Autodesk Inventor part; units mm, degrees
ref_plane "YZ Plane" through (0, 0, 0) normal (1, 0, 0) x (0, 1, 0)
ref_plane "XZ Plane" through (0, 0, 0) normal (0, 1, 0) x (-1, 0, 0)
ref_plane "XY Plane" through (0, 0, 0) normal (0, 0, 1) x (1, 0, 0)
sketch "スケッチ1" plane through (0, 0, 0) normal (0, 0, 1) x (1, 0, 0)
  line L0 (-25, -71.3) -> (25, -71.3)
  line L1 (25, -71.3) -> (25, 25)
  line L2 (25, 25) -> (-25, 25)
  line L3 (-25, 25) -> (-25, -71.3)
  line L4 (-25, -71.3) -> (25, 25) construction
  line L5 (25, -71.3) -> (-25, 25) construction
  circle A0 centre (0, 0) radius 19 construction
  point P0 (0, -23.15)
  point P1 (0, -23.15)
  dimension "d0" = 38
  dimension "d1" = 50
  dimension "d2" = 25
  dimension "d3" = 71.3
extrude "プレート1" add sketch "スケッチ1" along normal blind 2.3
sketch "スケッチ9" plane through (25, -69, 0) normal (0, -1, 0) x (1, 0, 0)
  line L0 (-50, 0) -> (0, 0)
  line L1 (0, 0) -> (0, 14.6)
  line L2 (0, 14.6) -> (-50, 14.6)
  line L3 (-50, 14.6) -> (-50, 0)
edge flange "フランジ3" height 14.6 angle 90 thickness 2.3 bend radius 2.3 thickness toward (0, -1, 0) relief tear relief width 2.3 relief depth 1.15 edges at (0, -71.3, 2.3) wall of the first edge with corners at (-25, -69, 0) (25, -69, 0) (25, -69, 14.6) (-25, -69, 14.6)
bend "曲げ3"
corner "コーナー3"
fillet "コーナーR1" radius 5 2 edges at (25, -70.15, 14.6) (-25, -70.15, 14.6)
sketch "スケッチ4" plane through (0, 0, 2.3) normal (0, 0, 1) x (1, 0, 0)
  circle A0 centre (0, 0) radius 15
  point P0 (0, 15)
  point P1 (-15, 0)
  point P2 (0, -15)
  point P3 (15, 0)
  dimension "d26" = 30
  dimension "d29" = 360
hole "穴1" at (0, 15, 2.3) at (-15, 0, 2.3) at (0, -15, 2.3) at (15, 0, 2.3) direction (0, 0, -1) diameter 3.2 end through all
sketch "スケッチ5" plane through (0, 0, 2.3) normal (0, 0, 1) x (1, 0, 0)
  circle A0 centre (0, 0) radius 16
  point P0 (-11.3137, 11.3137)
  point P1 (-11.3137, -11.3137)
  point P2 (11.3137, -11.3137)
  point P3 (11.3137, 11.3137)
  dimension "d38" = 32
  dimension "d41" = 360
hole "穴2" at (-11.3137, 11.3137, 2.3) at (-11.3137, -11.3137, 2.3) at (11.3137, -11.3137, 2.3) at (11.3137, 11.3137, 2.3) direction (0, 0, -1) diameter 4.3 end through all
sketch "スケッチ6" plane through (0, 0, 2.3) normal (0, 0, 1) x (1, 0, 0)
  circle A0 centre (0, 0) radius 10
  dimension "d50" = 20
extrude "押し出し1" cut sketch "スケッチ6" against normal blind 10
sketch "スケッチ7" plane through (-25, -69, -2.3) normal (0, 1, 0) x (1, 0, 0)
  line L0 (5, -16.9) -> (45, -16.9)
  line L1 (0, -6.9) -> (0, -11.9)
  line L2 (50, -6.9) -> (50, -11.9)
  point P0 (18, -2.3)
  point P1 (45, -11.9)
  point P2 (5, -11.9)
  dimension "d76" = 5
  dimension "d77" = 5
  dimension "d78" = 5
hole "穴3" at (20, -69, 9.6) at (-20, -69, 9.6) direction (0, -1, 0) diameter 4.3 end through all
fillet "コーナーR3" radius 10 2 edges at (-25, 25, 1.15) (25, 25, 1.15)
sketch "スケッチ10" plane through (0, 0, 0) normal (0, 0, -1) x (-1, 0, 0)
  line L0 (-25, -66.7) -> (-25, 15)
  line L1 (25, 15) -> (25, -66.7)
  circle A0 centre (-20, -44.5) radius 4
  circle A1 centre (0, 0) radius 45
  point P0 (20, -44.5)
  dimension "d80" = 5
  dimension "d81" = 5
  dimension "d82" = 44.5
  dimension "d83" = 8
  dimension "d84" = 90
hole "穴4" at (20, -44.5, 0) at (-20, -44.5, 0) direction (0, 0, 1) diameter 4.3 end through all
sketch "スケッチ11" plane through (0, 0, 2.3) normal (0, 0, 1) x (1, 0, 0)
  circle A0 centre (0, -36) radius 5
  point P0 (0, 0)
  dimension "d92" = 10
  dimension "d93" = 36
extrude "押し出し3" cut sketch "スケッチ11" against normal blind 10
equation "\"d36\" = Thickness"
equation "\"d48\" = Thickness"
equation "\"d61\" = Thickness"
equation "\"d90\" = Thickness"
equation "\"d4\" = Thickness"
equation "\"d66\" = BendReliefWidth"
equation "\"d67\" = BendReliefDepth"
equation "\"d68\" = MinimumRemnant"
equation "\"d69\" = TransitionRadius"
equation "\"d72\" = BendRadius"
equation "\"d73\" = CornerReliefSize"
equation "\"d74\" = GapSize"
equation "\"d75\" = JacobiRadiusSize"
equation "\"BendRadius\" = Thickness"
equation "\"BendReliefWidth\" = Thickness"
equation "\"BendReliefDepth\" = 0.5 * Thickness"
equation "\"CornerReliefSize\" = 4 * Thickness"
equation "\"MinimumRemnant\" = 2 * Thickness"
equation "\"TransitionRadius\" = BendRadius"
equation "\"JacobiRadiusSize\" = BendRadius"
equation "\"GapSize\" = Thickness"
properties part number "plate8" material "鋼、炭素鋼"
For this review, take the finished solid that the model builds, in its own axes (mm). A direction names the side the tool comes from. Give positions to 0.01 mm unless a question says otherwise; leave off trailing zeros. Loops run counter-clockwise (first coordinate to the right, second up) from the corner with the lowest first, then second, coordinate; pieces in that order, holes last. Notation, with made-up numbers: M 57,69.5 L 86,69.5 A14 cw 86,76.5 Z; hole C -22,9.5 d10. An arc over 180 degrees is marked long. One line per item, written item: value. Start each with the question number.
Q1. Clearance check with flat-ended pins moving along their axes: pin 1 Ø3.5 at (x, y) = (11.31, -11.31) entering from +Z; pin 2 Ø5 at (x, z) = (3, 9) entering from +Y; pin 3 Ø5 at (x, y) = (-7.5, -58) entering from +Z. State where each tip first meets the part, or that it passes through.
Q2. Add section C-C (x = -6). Give the boundary of the cut face in (y, z), and give its area (3 significant figures).
Q3. Add section B-B (y = 0). Give the boundary of the cut face in (x, z).
Q4. Add section D-D (z = 5.5). Give the boundary of the cut face in (x, y).
Q5. Add section A-A (y = -15). Give the boundary of the cut face in (x, z).
Q6. For L1, parallel to X at y = -44.5, z = 1.75; L2, parallel to Y at x = 1, z = 1; L3, parallel to Y at x = 0, z = 1.4, list the stretches that pass through material, from the lowest coordinate up.
Q7. Machinability: for faces 1 (the face through (0, -69, 10)), 2 (the face through (0, -71.3, 10)), which of the approach directions +Z, -Z, +X, -X, +Y, -Y give a long, thin tool a straight path to every point of the face, cutting with its end or side? Answer none if there is none.
Q8. Draft analysis for pull direction Y (two halves, no side actions). For faces 3 (the face through (0.35, -69.988, 1.383)), 4 (the face through (-10.005, -9.608, 1.134)), 5 (the face through (22.1, -70.17, 9.13)), state which applies: released by +Y, released by -Y, zero draft, split by the parting line, or undercut.
Reply:
1. pin 1: through
1. pin 2: y = -69
1. pin 3: z = 2.3
2. outline: M -71.3,4.6 A4.6 ccw -66.7,0 L -8,0 L -8,2.3 L -66.7,2.3 A2.3 cw -69,4.6 L -69,14.6 L -71.3,14.6 Z; M 8,0 L 25,0 L 25,2.3 L 8,2.3 Z
2. area: 210 mm²
3. outline: M -25,0 L -16.6,0 L -16.6,2.3 L -25,2.3 Z; M -13.4,0 L -10,0 L -10,2.3 L -13.4,2.3 Z; M 10,0 L 13.4,0 L 13.4,2.3 L 10,2.3 Z; M 16.6,0 L 25,0 L 25,2.3 L 16.6,2.3 Z
4. outline: M -25,-71.3 L 25,-71.3 L 25,-69 L -25,-69 Z
5. outline: M -25,0 L -1.6,0 L -1.6,2.3 L -25,2.3 Z; M 1.6,0 L 25,0 L 25,2.3 L 1.6,2.3 Z
6. L1: -25 to -22.15, -17.85 to 17.85, 22.15 to 25
6. L2: -69.56 to -40.9, -31.1 to -16.25, -13.75 to -9.95, 9.95 to 13.75, 16.25 to 25
6. L3: -70 to -41, -31 to -16.6, -13.4 to -10, 10 to 13.4, 16.6 to 25
7. face 1: +Z, +X, -X, +Y
7. face 2: +Z, -Z, +X, -X, -Y
8. face 3: released by -Y
8. face 4: undercut
8. face 5: zero draft
